```python
from build123d import *

# Parameters (mm, degrees)
RESSALTO_EXTRUS_O1_DEPTH   = 15
FURO_DE_DI_METRO_7_0_7_1_D = 7


with BuildPart() as part:
    # Esboço1 → Ressalto-extrusão1 (new body, symmetric)
    with BuildSketch(Plane.XY):
        with BuildLine():
            Line((15, 0), (37.5, 0))
            Line((37.5, 0), (37.5, 6))
            Line((37.5, 6), (20.124611797, 6))
            ThreePointArc((20.124611797, 6), (0, 21), (-20.124611797, 6))
            Line((-20.124611797, 6), (-37.5, 6))
            Line((-37.5, 6), (-37.5, 0))
            Line((-37.5, 0), (-15, 0))
            ThreePointArc((-15, 0), (0, 15), (15, 0))
        make_face()
    extrude(amount=RESSALTO_EXTRUS_O1_DEPTH, both=True)

    # Furo de diâmetro Ø7.0 (7)1 (through all)
    with Locations(Plane(origin=(0, 6, 0), x_dir=(1, 0, 0), z_dir=(0, 1, 0))):
        with Locations((-28.75, 0), (28.75, 0)):
            Hole(FURO_DE_DI_METRO_7_0_7_1_D / 2)


solid = part.part
```
Could you check a few things on this model? Use its own coordinates, in mm. A direction names the side the tool comes from. Round coordinates to 2 decimals unless told otherwise and drop trailing zeros. Loops run counter-clockwise (first coordinate to the right, second up) from the corner with the lowest first, then second, coordinate; pieces in that order, holes last. Notation, with made-up numbers: (-4.75, 67) -> (36.25, 67) arc R14 cw to (36.25, 91) -> close; hole circle Ø3 at (15.25, -3). An arc over 180 degrees is marked (long way). One line per question, with ' | ' between items.
(1) If we section it at B-B on x = 28.75: List the corners of the cut face in (y, z) for me, and give its area (3 significant figures).
Model answer:
outline: (0, -15) -> (6, -15) -> (6, -3.5) -> (0, -3.5) -> close; (0, 3.5) -> (6, 3.5) -> (6, 15) -> (0, 15) -> close | area: 138 mm^2
(2) If we section it at A-A on z = 0: List the corners of the cut face in (x, y) for me, and give its area (3 significant figures).
Model answer:
outline: (-37.5, 0) -> (-32.25, 0) -> (-32.25, 6) -> (-37.5, 6) -> close; (-25.25, 0) -> (-15, 0) arc R15 cw to (15, 0) -> (25.25, 0) -> (25.25, 6) -> (20.12, 6) arc R21 ccw to (-20.12, 6) -> (-25.25, 6) -> close; (32.25, 0) -> (37.5, 0) -> (37.5, 6) -> (32.25, 6) -> close | area: 457 mm^2
(3) If I drill on probe 1 along Z at (x, y) = (-28.75, 2.35); probe 2 along X at (y, z) = (5.5, -2.25); probe 3 along X at (y, z) = (4.75, -5.5), over which ranges is the centre line in solid material (lowest first)?
Model answer:
probe 1: z = -15 to -3.5, 3.5 to 15 | probe 2: x = -37.5 to -31.43, -26.07 to -13.96, 13.96 to 26.07, 31.43 to 37.5 | probe 3: x = -37.5 to -14.23, 14.23 to 37.5
(4) For faces 1 (the face through (29, 6, 4)), 2 (the face through (-37.5, 3, 0)), 3 (the face through (-29, 6, 4)), which set-ups out of +Z, -Z, +X, -X, +Y, -Y let a thin tool reach every point of the face, with its end or its side?
Model answer:
face 1: +Z, -Z, +X, +Y | face 2: +Z, -Z, -X, +Y, -Y | face 3: +Z, -Z, -X, +Y
(5) Thinking about a two-plate mould opening in X: for faces 4 (the face through (37.5, 3, 0)), 5 (the face through (25.41, 2.96, -1.05)), 6 (the face through (-32.09, 2.96, -1.05)), 7 (the face through (-0.5, 15.3, 15)), which applies, released by +X, released by -X, zero draft, split by the parting line, or undercut?
Model answer:
face 4: released by +X | face 5: undercut | face 6: undercut | face 7: zero draft
(6) If we section it at D-D on z = 5.25: List the corners of the cut face in (x, y) for me, and give its area (3 significant figures).
Model answer:
outline: (-37.5, 0) -> (-15, 0) arc R15 cw to (15, 0) -> (37.5, 0) -> (37.5, 6) -> (20.12, 6) arc R21 ccw to (-20.12, 6) -> (-37.5, 6) -> close | area: 541 mm^2
(7) If we section it at C-C on y = 1.75: List the corners of the cut face in (x, z) for me.
Model answer:
outline: (-37.5, -15) -> (-14.9, -15) -> (-14.9, 15) -> (-37.5, 15) -> close; (14.9, -15) -> (37.5, -15) -> (37.5, 15) -> (14.9, 15) -> close; hole circle Ø7 at (-28.75, 0); hole circle Ø7 at (28.75, 0)
(8) For pin 1 Ø2 at (y, z) = (13.5, -9) entering from -X; pin 2 Ø14 at (x, z) = (29, 2.5) entering from +Y; pin 3 Ø6 at (y, z) = (12.5, 4.5) entering from +X, each with a flat end and sliding along its axis, tell me the tip position at first contact or that it passes through.
Model answer:
pin 1: stops at x = -16.87 | pin 2: stops at y = 6 | pin 3: stops at x = 18.73
